```python
from build123d import *

# Parameters (mm, degrees)
F0_R     = 38.1
F1_DEPTH = 47.625
F2_R     = 50.8
F3_DEPTH = 3.175
F4_R     = 12.7
F5_DEPTH = 47.625
F6_DEPTH = 3.175


with BuildPart() as f1:
    # F0 (on Front) → F1 (new body)
    with BuildSketch(Plane.XZ):
        Circle(F0_R)
    extrude(amount=F1_DEPTH)

    # F2 (on Front) → F3 (join)
    with BuildSketch(Plane.XZ):
        with Locations((3.468244, 0)):
            Circle(F2_R)
    extrude(amount=-F3_DEPTH)

    # F4 (on Front) → F5 (cut, through all)
    with BuildSketch(Plane.XZ):
        Circle(F4_R)
    extrude(amount=F5_DEPTH, mode=Mode.SUBTRACT)

    # F4 (on Front) → F6 (cut, through all)
    with BuildSketch(Plane.XZ):
        Circle(F4_R)
    extrude(amount=-F6_DEPTH, mode=Mode.SUBTRACT)


solid = f1.part
```
Could you check a few things on this model? Use its own coordinates, in mm. A direction names the side the tool comes from. Round coordinates to 2 decimals unless told otherwise and drop trailing zeros. Loops run counter-clockwise (first coordinate to the right, second up) from the corner with the lowest first, then second, coordinate; pieces in that order, holes last. Notation, with made-up numbers: (-28, 0.5) - (-4, 0.5) arc R16 cw to (-4, 9.5) - close; hole circle Ø1 at (19, -36). An arc over 180 degrees is marked (long way). Answer in a Markdown table with one row per item. Add a question column.
(1) If we section it at B-B (x = 0): Please give me the cut outline in (y, z) (3 decimals), plus the area to 3 significant figures.
(2) I'm going to push flat-ended pins straight in: pin 1 (3 mm diameter, centred on y = -41, z = 12.5, fed in from +X); pin 2 (12 mm diameter, centred on x = -13.5, y = -38, fed in from +Z); pin 3 (6 mm diameter, centred on x = -9.5, y = -28, fed in from -Z); pin 4 (15 mm diameter, centred on x = 0, z = 0, fed in from -Y). Where does each tip first touch, or does it pass through?
(3) For faces 1 (the face through (37, 0, -11)), 2 (the face through (16, -47.625, 1)), which set-ups out of +Z, -Z, +X, -X, +Y, -Y let a thin tool reach every point of the face, with its end or its side?
(4) If we section it at C-C (x = -25): Please give me the cut outline in (y, z) (3 decimals), plus the area to 3 significant figures.
(5) If we section it at A-A (z = 0): Please give me the cut outline in (x, y) (3 decimals).
(6) I need wall thicknesses on line 1 along Z through (x, y) = (0, -11); line 2 along Y through (x, z) = (47.5, -10.5) (3 decimals); line 3 along Z through (x, y) = (0, 2.4). Which ranges of each line are inside material? Lowest first, please.
(7) If we section it at D-D (y = -3): Please give me the cut outline in (x, z).
Model answer:
| question | item | result |
|---|---|---|
| 1 | outline | (-47.625, -38.1) - (0, -38.1) - (0, -50.681) - (3.175, -50.681) - (3.175, -12.7) - (-47.625, -12.7) - close; (-47.625, 12.7) - (3.175, 12.7) - (3.175, 50.681) - (0, 50.681) - (0, 38.1) - (-47.625, 38.1) - close |
| 1 | area | 2,660 mm² |
| 2 | pin 1 | stops at x = 36.48 |
| 2 | pin 2 | stops at z = 37.35 |
| 2 | pin 3 | stops at z = -37.54 |
| 2 | pin 4 | passes through |
| 3 | face 1 | -Y |
| 3 | face 2 | +Z, -Z, +X, -X, -Y |
| 4 | outline | (-47.625, -28.751) - (0, -28.751) - (0, -42.074) - (3.175, -42.074) - (3.175, 42.074) - (0, 42.074) - (0, 28.751) - (-47.625, 28.751) - close |
| 4 | area | 3,010 mm² |
| 5 | outline | (-47.332, 0) - (-38.1, 0) - (-38.1, -47.625) - (-12.7, -47.625) - (-12.7, 3.175) - (-47.332, 3.175) - close; (12.7, -47.625) - (38.1, -47.625) - (38.1, 0) - (54.268, 0) - (54.268, 3.175) - (12.7, 3.175) - close |
| 6 | line 1 | z = -38.1 to -12.7, 12.7 to 38.1 |
| 6 | line 2 | y = 0 to 3.175 |
| 6 | line 3 | z = -50.68 to -12.7, 12.7 to 50.68 |
| 7 | outline | circle Ø76.2 at (0, 0); hole circle Ø25.4 at (0, 0) |
